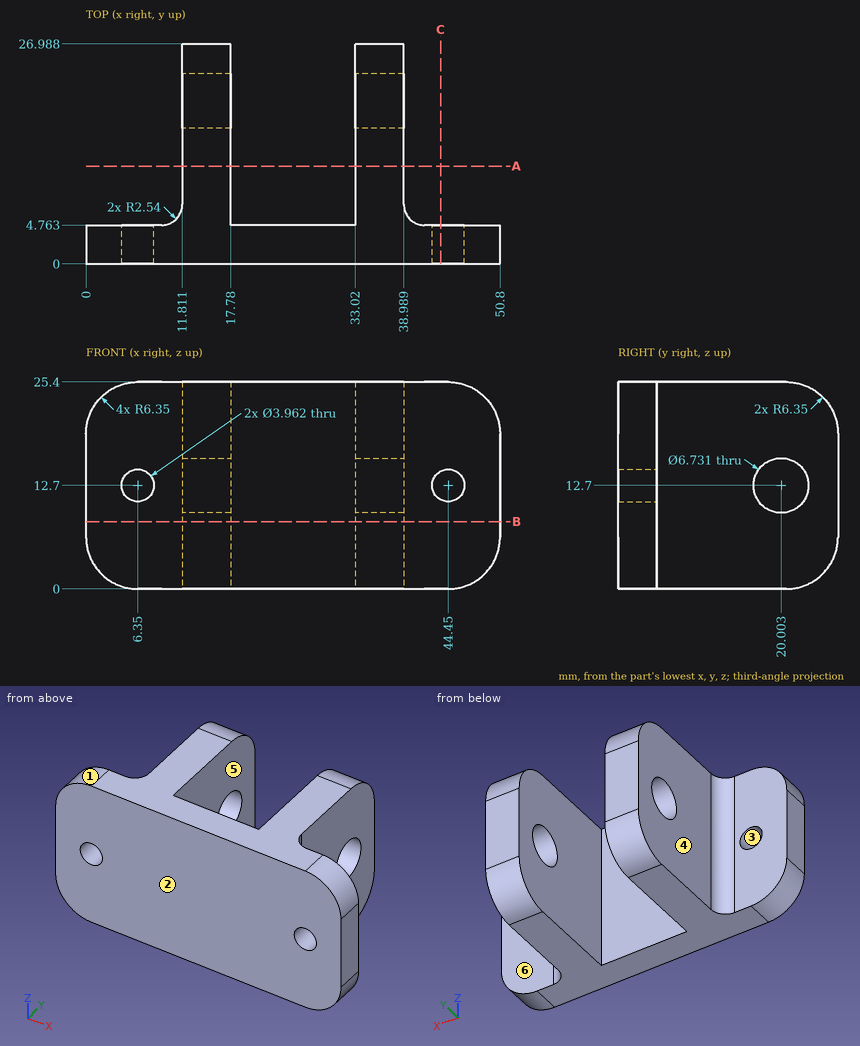
Answer from the drawing. Dimensions are ordinates in mm from the lowest x, y and z of the part. A direction names the side the tool comes from. Give positions to 0.01 mm unless a question says otherwise; leave off trailing zeros. Order: outer loops, then holes, each group sorted by start corner. A loop starts at its lowest first (then second) coordinate and runs counter-clockwise, first axis right, second up. Notation, with made-up numbers: (-6.5, 77) - (48.5, 77) arc R25 ccw to (48.5, 102) - close; hole circle Ø11 at (67, -1.5). An arc over 180 degrees is marked (long way). Use one line per item in the form item = value.
1) Consider probe 1 along X at (y, z) = (3.65, 12.7); probe 2 along X at (y, z) = (20.25, 20.5); probe 3 along Y at (x, z) = (36.1, 12.7). Determine where each line is inside the solid, lowest interval first. Write a range as [from, to].
Verdict:
probe_1 = [0, 4.37], [8.33, 42.47], [46.43, 50.8]
probe_2 = [11.81, 17.78], [33.02, 38.99]
probe_3 = [0, 16.64], [23.37, 26.99]
2) For the marked faces 4, 5 and 6, determine the directions among +Z, -Z, +X, -X, +Y, -Y from which every point of the face is accessible in a straight line to the end or side of a thin tool.
Verdict:
face_4 = +Z, -Z, -X, +Y
face_5 = +Z, -Z, +Y
face_6 = +Z, -Z, +X, +Y
3) Find section C-C on x = 43.5. Determine the outline of the cut face in (y, z), and give its area (3 significant figures).
Verdict:
outline = (0, 0) - (4.76, 0) - (4.76, 10.96) - (0, 10.96) - close; (0, 14.44) - (4.76, 14.44) - (4.76, 25.4) - (0, 25.4) - close
area = 104 mm^2
4) Each of these flat-tipped pins is pushed along its axis until it touches: pin 1 (3 mm diameter, centred on x = 6.5, z = 9.5, fed in from +Y); pin 2 (2 mm diameter, centred on y = 6, z = 21, fed in from -X) (1 decimal); pin 3 (6.5 mm diameter, centred on y = 21, z = 12, fed in from -X); pin 4 (2.5 mm diameter, centred on x = 44.45, z = 12.7, fed in from +Y). Where does it stop, or does it pass through?
Verdict:
pin_1 = 4.76
pin_2 = 10.3
pin_3 = 11.81
pin_4 = through
5) Find section A-A on y = 12. Determine the outline of the cut face in (x, z).
Verdict:
outline = (11.81, 0) - (17.78, 0) - (17.78, 25.4) - (11.81, 25.4) - close; (33.02, 0) - (38.99, 0) - (38.99, 25.4) - (33.02, 25.4) - close
6) The mould has two halves that part along Z. Classify the marked faces 1, 2 and 3: released by +Z, released by -Z, zero draft, split by the parting line, or undercut.
Verdict:
face_1 = released by +Z
face_2 = zero draft
face_3 = undercut
7) Find section B-B on z = 8.25. Determine the outline of the cut face in (x, y).
Verdict:
outline = (0, 0) - (50.8, 0) - (50.8, 4.76) - (41.53, 4.76) arc R2.54 cw to (38.99, 7.3) - (38.99, 26.99) - (33.02, 26.99) - (33.02, 4.76) - (17.78, 4.76) - (17.78, 26.99) - (11.81, 26.99) - (11.81, 7.3) arc R2.54 cw to (9.27, 4.76) - (0, 4.76) - close
